Input: part model. Units: mm. Frame: model coordinates. Coordinates: 2 decimals unless noted, no trailing zeros. Loops run counter-clockwise (first coordinate to the right, second up) from the corner with the lowest first, then second, coordinate; pieces in that order, holes last. Notation, with made-up numbers: (38, -21) -> (80, -21) arc R29 ccw to (80, 16) -> close; hole circle Ø3 at (7.5, 16.25). An arc over 180 degrees is marked (long way). Answer as a JSON object with one key per item and string values.
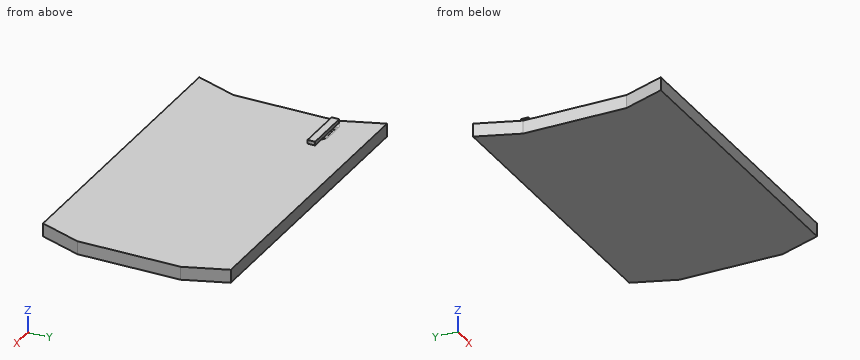
Autodesk Inventor part; units mm, degrees
ref_plane "YZ Plane" through (0, 0, 0) normal (1, 0, 0) x (0, 1, 0)
ref_plane "XZ Plane" through (0, 0, 0) normal (0, 1, 0) x (-1, 0, 0)
ref_plane "XY Plane" through (0, 0, 0) normal (0, 0, 1) x (1, 0, 0)
sketch "Эскиз1" plane through (0, 0, 0) normal (0, 0, 1) x (1, 0, 0)
  line L0 (0, 0) -> (170, 0)
  line L1 (170, 0) -> (170, 100)
  line L2 (170, 100) -> (0, 100)
  line L3 (0, 100) -> (0, 0) construction
  line L4 (0, 100) -> (8.1893, 77.5)
  line L5 (8.1893, 77.5) -> (8.1893, 22.5)
  line L6 (8.1893, 22.5) -> (0, 0)
  line L7 (161.8107, 100) -> (170, 77.5)
  line L8 (170, 22.5) -> (161.8107, 0)
  dimension "d0" = 170
  dimension "d1" = 100
  dimension "d2" = 20
  dimension "d3" = 55
  dimension "d4" = 20
  dimension "d6" = 55
  dimension "d7" = 20
extrude "Выдавливание1" add sketch "Эскиз1" against normal blind 7 contours L6 L5 L4 L2 L7 L1 L8 L0
sketch "Эскиз2" plane through (0, 0, 0) normal (0, 0, 1) x (1, 0, 0)
  line L0 (14.0981, 75.5) -> (25.0981, 75.5)
  line L1 (27.0981, 77.5) -> (27.0981, 77.5)
  line L2 (25.0981, 79.5) -> (14.0981, 79.5)
  line L3 (12.0981, 77.5) -> (12.0981, 77.5)
  line L4 (12.0981, 75.5) -> (27.0981, 79.5) construction
  line L5 (27.0981, 75.5) -> (12.0981, 79.5) construction
  arc A0 (14.0981, 79.5) -> (12.0981, 77.5) centre (14.0981, 77.5) ccw
  arc A1 (12.0981, 77.5) -> (14.0981, 75.5) centre (14.0981, 77.5) ccw
  arc A2 (25.0981, 75.5) -> (27.0981, 77.5) centre (25.0981, 77.5) ccw
  arc A3 (27.0981, 77.5) -> (25.0981, 79.5) centre (25.0981, 77.5) ccw
  point P0 (0, 0)
  point P1 (19.5981, 77.5)
  dimension "d10" = 15
  dimension "d11" = 4
  dimension "d12" = 2
extrude "Выдавливание2" cut sketch "Эскиз2" against normal blind 2
fillet "Сопряжение1" radius 2 4 edges at (27.0981, 77.5, 0) (19.5981, 75.5, 0) (12.0981, 77.5, 0) (19.5981, 79.5, 0)
fillet "Сопряжение2" radius 2 8 edges at (19.5981, 79.5, -1.9995) (19.5981, 79.5, -2) (27.0981, 77.5, -1.9995) (27.0981, 77.5, -2) (19.5981, 75.5, -1.9995) (19.5981, 75.5, -2) (12.0981, 77.5, -1.9995) (12.0981, 77.5, -2)
sketch "Эскиз3" plane through (0, 0, 0) normal (0, 0, 1) x (1, 0, 0)
  line L0 (9.6893, 79.5) -> (34.6893, 79.5)
  line L1 (34.6893, 79.5) -> (34.6893, 75.5)
  line L2 (34.6893, 75.5) -> (9.6893, 75.5)
  line L3 (9.6893, 75.5) -> (9.6893, 79.5)
  line L4 (14.0981, 73.5) -> (25.0981, 73.5)
  line L5 (8.1893, 77.5) -> (8.1893, 22.5)
  point P0 (0, 0)
  dimension "d17" = 4
  dimension "d18" = 25
  dimension "d19" = 2
  dimension "d20" = 1.5
extrude "Выдавливание3" add sketch "Эскиз3" along normal blind 2
properties part number "ДИ 00.00.03"
1. Line query: line 1 along Z through (x, y) = (148, 25.5); line 2 along X through (y, z) = (49.5, -4.75); line 3 along X through (y, z) = (7.5, -5.25). Output: solid intervals per line, ascending.
Reply:
{"line 1": "z = -7 to 0", "line 2": "x = 8.19 to 170", "line 3": "x = 2.73 to 164.54"}
2. Section query C-C (y = 18). Return loops of the section in (x, z).
Reply:
{"outline": "(6.55, -7) -> (168.36, -7) -> (168.36, 0) -> (6.55, 0) -> close"}
3. Section query B-B (x = 154). Return loops of the section in (y, z), plus the area to 3 significant figures.
Reply:
{"outline": "(0, -7) -> (100, -7) -> (100, 0) -> (0, 0) -> close", "area": "700 mm2"}
4. Section query A-A (z = -3.75). Return loops of the section in (x, y), plus the area to 3 significant figures.
Reply:
{"outline": "(0, 0) -> (161.81, 0) -> (170, 22.5) -> (170, 77.5) -> (161.81, 100) -> (0, 100) -> (8.19, 77.5) -> (8.19, 22.5) -> close", "area": "16,200 mm2"}
5. Pin query (flat end, axial travel): P1, Ø1, axis at y = 10.5, z = -4, coming from the +X side; P2, Ø1.6, axis at x = 24, z = 1, coming from the +Y side; P3, Ø1, axis at x = 22, z = 1, coming from the -Y side; P4, Ø6, axis at x = 33.5, y = 75, coming from the +Z side. Return the tip coordinate at first contact, or that it passes through.
Reply:
{"P1": "stops at x = 165.81", "P2": "stops at y = 79.5", "P3": "stops at y = 75.5", "P4": "stops at z = 2"}
